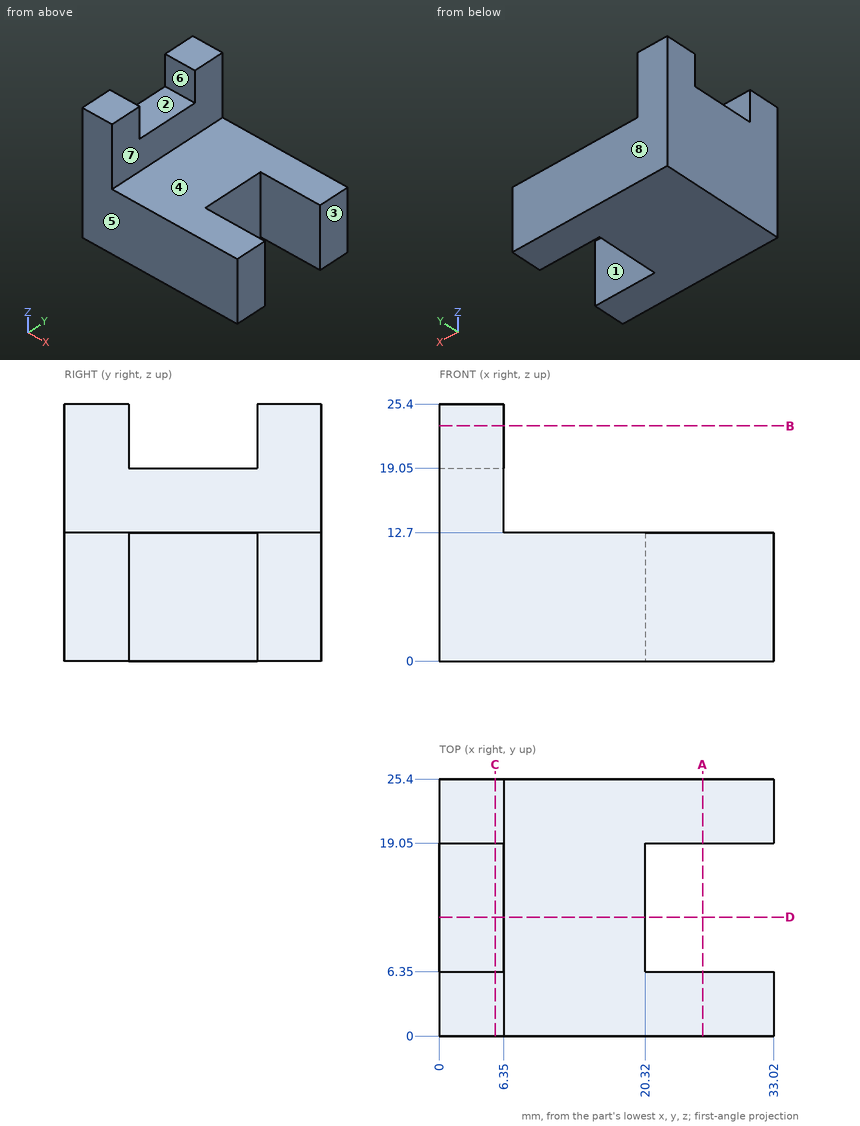
Check sheet for the drawn part. Datum: minimum x, y, z corner. Units: mm. A direction names the side the tool comes from. Round coordinates to 2 decimals unless told otherwise and drop trailing zeros. Loops run counter-clockwise (first coordinate to the right, second up) from the corner with the lowest first, then second, coordinate; pieces in that order, holes last. Notation, with made-up numbers: M 25,13 L 82,13 A14 ccw 82,26 Z; hole C 25.5,-18.75 d3. An arc over 180 degrees is marked long. One line per question, with ' | ' between items. Start each with the question number.
Item 1: Set-up check for the marked faces 1, 2, 3, 4 and 5: record each of +Z, -Z, +X, -X, +Y, -Y from which the full face is reachable in a straight line by a thin tool's end or side.
Item 2: Section check D-D (y = 11.75). Record the boundary of the cut face in (x, z), and give its area (3 significant figures).
Item 3: Release check for a two-part mould opening along Y. For the marked faces 6, 7 and 8 record: released by +Y, released by -Y, zero draft, split by the parting line, or undercut.
Item 4: Scan lines: probe 1 along Y at (x, z) = (28.5, 5.5); probe 2 along X at (y, z) = (13.25, 13.75); probe 3 along X at (y, z) = (10.5, 11.5). Record each from-to range of solid material in increasing order.
Item 5: Section check C-C (x = 5.5). Record the boundary of the cut face in (y, z).
Item 6: Section check B-B (z = 23.25). Record the boundary of the cut face in (x, y), and give its area (3 significant figures).
Item 7: Gauge pin test, flat ends, axial feed: pin 1 Ø6.5 at (y, z) = (16.5, 17.5) entering from +X; pin 2 Ø1 at (x, y) = (11, 22) entering from +Z; pin 3 Ø1.5 at (y, z) = (8, 7) entering from +X. Record the tip position at first contact, or that the pin passes through.
Item 8: Section check A-A (x = 26). Record the boundary of the cut face in (y, z).
Worked out:
1) face 1: +Z, -Z, +X | face 2: +Z, +X, -X | face 3: +Z, -Z, +X, +Y, -Y | face 4: +Z, +X, +Y, -Y | face 5: +Z, -Z, +X, -X, -Y
2) outline: M 0,0 L 20.32,0 L 20.32,12.7 L 6.35,12.7 L 6.35,19.05 L 0,19.05 Z | area: 298 mm^2
3) face 6: undercut | face 7: zero draft | face 8: released by +Y
4) probe 1: 0 to 6.35, 19.05 to 25.4 | probe 2: 0 to 6.35 | probe 3: 0 to 20.32
5) outline: M 0,0 L 25.4,0 L 25.4,25.4 L 19.05,25.4 L 19.05,19.05 L 6.35,19.05 L 6.35,25.4 L 0,25.4 Z
6) outline: M 0,0 L 6.35,0 L 6.35,6.35 L 0,6.35 Z; M 0,19.05 L 6.35,19.05 L 6.35,25.4 L 0,25.4 Z | area: 80.6 mm^2
7) pin 1: x = 6.35 | pin 2: z = 12.7 | pin 3: x = 20.32
8) outline: M 0,0 L 6.35,0 L 6.35,12.7 L 0,12.7 Z; M 19.05,0 L 25.4,0 L 25.4,12.7 L 19.05,12.7 Z
